Check sheet for the modelled part. Datum: model origin and axes. Units: mm. Round coordinates to 2 decimals unless told otherwise and drop trailing zeros. Loops run counter-clockwise (first coordinate to the right, second up) from the corner with the lowest first, then second, coordinate; pieces in that order, holes last. Notation, with made-up numbers: (74, 8.5) - (96, 8.5) arc R26 cw to (96, 47.5) - close; hole circle Ø7 at (-16, 50). An arc over 180 degrees is marked (long way). Answer in a Markdown table with one row per item. Add a question column.
(1) Cross-section at C-C on z = 1.65. Enter the section's corners in (x, y), then the cut area to 3 significant figures.
(2) Cross-section at D-D on y = 0. Enter the section's corners in (x, z), then the cut area to 3 significant figures.
(3) Cross-section at A-A on x = -20. Enter the section's corners in (y, z).
(4) Thickness scan on line 1 along Y through (x, z) = (-20, 3.85); line 2 along Y through (x, z) = (0, 0.45); line 3 along X through (y, z) = (19.5, 2.95). Record the ranges inside material, lowest first.
(5) Mould release check, pull along Y, two halves, no side actions. Record for faces 1 (the flat face through (0, 25, 2)), 2 (the flat face through (25, 0, 2)), 3 (the cylindrical face through (5.96, 1.88, 2.97)), 4 (the flat face through (-1.3, -4.1, 1)): +Y half, -Y half, draft (parallel to the pull), parting line (faces both ways), or undercut.
(6) Gauge pin test, flat end, axial feed: pin 1 (5.5 mm diameter, centred on x = -20, y = 20, fed in from +Z). Record the tip position at first contact, or that the pin passes through.
from build123d import *

# Parameters (mm, degrees)
SKETCH_1_W      = 50
SKETCH_1_H      = 50
SKETCH_1_R      = 1.65
SKETCH_1_R_2    = 6.25
EXTRUDE_1_DEPTH = 5
SKETCH_2_R      = 6.25
SKETCH_2_R_2    = 4
EXTRUDE_2_DEPTH = 1


with BuildPart() as part:
    # 草图1 → 凸台-拉伸1 (new body)
    with BuildSketch(Plane.XY):
        Rectangle(SKETCH_1_W, SKETCH_1_H)
        with Locations((-20, -20)):
            Circle(SKETCH_1_R, mode=Mode.SUBTRACT)
        with Locations((-20, 20)):
            Circle(SKETCH_1_R, mode=Mode.SUBTRACT)
        with Locations((20, 20)):
            Circle(SKETCH_1_R, mode=Mode.SUBTRACT)
        with Locations((20, -20)):
            Circle(SKETCH_1_R, mode=Mode.SUBTRACT)
        Circle(SKETCH_1_R_2, mode=Mode.SUBTRACT)
    extrude(amount=EXTRUDE_1_DEPTH)

    # 草图2 → 凸台-拉伸2 (add)
    with BuildSketch(Plane(origin=(0, 0, 0), x_dir=(-1, 0, 0), z_dir=(0, 0, -1))):
        Circle(SKETCH_2_R)
        Circle(SKETCH_2_R_2, mode=Mode.SUBTRACT)
    extrude(amount=-EXTRUDE_2_DEPTH)


solid = part.part
Answers:
| question | item | result |
|---|---|---|
| 1 | outline | (-25, -25) - (25, -25) - (25, 25) - (-25, 25) - close; hole circle Ø3.3 at (-20, -20); hole circle Ø3.3 at (-20, 20); hole circle Ø12.5 at (0, 0); hole circle Ø3.3 at (20, -20); hole circle Ø3.3 at (20, 20) |
| 1 | area | 2,340 mm^2 |
| 2 | outline | (-25, 0) - (-4, 0) - (-4, 1) - (-6.25, 1) - (-6.25, 5) - (-25, 5) - close; (4, 0) - (25, 0) - (25, 5) - (6.25, 5) - (6.25, 1) - (4, 1) - close |
| 2 | area | 192 mm^2 |
| 3 | outline | (-25, 0) - (-21.65, 0) - (-21.65, 5) - (-25, 5) - close; (-18.35, 0) - (18.35, 0) - (18.35, 5) - (-18.35, 5) - close; (21.65, 0) - (25, 0) - (25, 5) - (21.65, 5) - close |
| 4 | line 1 | y = -25 to -21.65, -18.35 to 18.35, 21.65 to 25 |
| 4 | line 2 | y = -25 to -4, 4 to 25 |
| 4 | line 3 | x = -25 to -21.57, -18.43 to 18.43, 21.57 to 25 |
| 5 | face 1 | +Y half |
| 5 | face 2 | draft |
| 5 | face 3 | undercut |
| 5 | face 4 | undercut |
| 6 | pin 1 | stops at z = 5 |
